Model file for the job. Use its own axes, mm. Face numbers are marked on the shaded views. A direction names the side the tool comes from. Round coordinates to 2 decimals unless told otherwise and drop trailing zeros. Order: outer loops, then holes, each group sorted by start corner. A loop starts at its lowest first (then second) coordinate and runs counter-clockwise, first axis right, second up. Notation, with made-up numbers: (6, -6.75) -> (52, -6.75) arc R29 cw to (52, 20.25) -> close; hole circle Ø8 at (-5.75, 12). An arc over 180 degrees is marked (long way). Put each result on its own line as item: value. Start each with the question number.
Q1. Cut at D-D, the plane z = 5. List the corners of the cut face in (x, y), and give its area (3 significant figures).
Q2. Cut at A-A, the plane z = 0. List the corners of the cut face in (x, y), and give its area (4 significant figures).
Q3. Flat gauge pins, fed straight in: P1, Ø5, axis at x = -10, z = 1.5, coming from the -Y side; P2, Ø2, axis at x = -5, z = 1.5, coming from the +Y side; P3, Ø4, axis at x = -18, y = -1, coming from the -Z side. Where does each tip first touch, or does it go through?
Q4. Probe L1, parallel to X at y = -4.25, z = -1.5; L2, parallel to X at y = -1.5, z = -3; L3, parallel to Y at x = -9.5, z = -1. List the from-to ranges inside material, lowest first.
Q5. Cut at C-C, the plane x = -6. List the corners of the cut face in (y, z).
Q6. Cut at B-B, the plane y = 0. List the corners of the cut face in (x, z), and give its area (4 significant figures).
Q7. 3-axis set-ups, long thin cutter, end or side, ignore diameter. For the marked faces 1 and 2: which of +Z, -Z, +X, -X, +Y, -Y reach the whole face in a straight line?
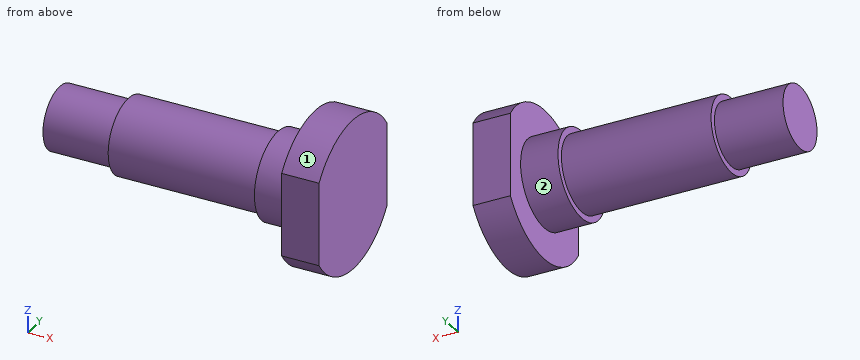
from build123d import *

# Parameters (mm, degrees)
BOSS_EXTRUDE1_DEPTH = 3
BOSS_EXTRUDE2_DEPTH = 15
BOSS_EXTRUDE3_DEPTH = 20.5
BOSS_EXTRUDE4_DEPTH = 3


with BuildPart() as part:
    # Sketch2 → Boss-Extrude1 (new body)
    with BuildSketch(Plane(origin=(0, 0, 0), x_dir=(0, 0, -1), z_dir=(1, 0, 0))):
        with BuildLine():
            Line((-3.31662479, 5), (3.31662479, 5))
            ThreePointArc((3.31662479, 5), (6, 0), (3.31662479, -5))
            Line((3.31662479, -5), (-3.31662479, -5))
            ThreePointArc((-3.31662479, -5), (-6, 0), (-3.31662479, 5))
        make_face()
    extrude(amount=BOSS_EXTRUDE1_DEPTH)

    # Sketch2_4 → Boss-Extrude2 (add)
    # profile 1 of 2: a face of its own
    with BuildSketch(Plane(origin=(0, 0, 0), x_dir=(0, 0, -1), z_dir=(1, 0, 0))):
        with BuildLine():
            ThreePointArc((3, 0), (0, 3), (-3, 0))
            ThreePointArc((-3, 0), (0, -3), (3, 0))
        make_face()
        with BuildLine():
            ThreePointArc((2.5, 0), (0, -2.5), (-2.5, 0))
            ThreePointArc((-2.5, 0), (0, 2.5), (2.5, 0))
        make_face(mode=Mode.SUBTRACT)
    # profile 2 of 2: a face of its own
    with BuildSketch(Plane(origin=(0, 0, 0), x_dir=(0, 0, -1), z_dir=(1, 0, 0))):
        with BuildLine():
            ThreePointArc((3, 0), (0, 3), (-3, 0))
            ThreePointArc((-3, 0), (0, -3), (3, 0))
        make_face()
        with BuildLine():
            ThreePointArc((2.5, 0), (0, -2.5), (-2.5, 0))
            ThreePointArc((-2.5, 0), (0, 2.5), (2.5, 0))
        make_face(mode=Mode.SUBTRACT)
    extrude(amount=-BOSS_EXTRUDE2_DEPTH)

    # Sketch2_5 → Boss-Extrude3 (add)
    with BuildSketch(Plane(origin=(0, 0, 0), x_dir=(0, 0, -1), z_dir=(1, 0, 0))):
        with BuildLine():
            ThreePointArc((2.5, 0), (0, 2.5), (-2.5, 0))
            ThreePointArc((-2.5, 0), (0, -2.5), (2.5, 0))
        make_face()
    extrude(amount=-BOSS_EXTRUDE3_DEPTH)

    # Sketch2_6 → Boss-Extrude4 (add)
    # profile 1 of 2: a face of its own
    with BuildSketch(Plane(origin=(0, 0, 0), x_dir=(0, 0, -1), z_dir=(1, 0, 0))):
        with BuildLine():
            ThreePointArc((3.5, 0), (0, 3.5), (-3.5, 0))
            ThreePointArc((-3.5, 0), (0, -3.5), (3.5, 0))
        make_face()
        with BuildLine():
            ThreePointArc((3, 0), (0, -3), (-3, 0))
            ThreePointArc((-3, 0), (0, 3), (3, 0))
        make_face(mode=Mode.SUBTRACT)
    # profile 2 of 2: a face of its own
    with BuildSketch(Plane(origin=(0, 0, 0), x_dir=(0, 0, -1), z_dir=(1, 0, 0))):
        with BuildLine():
            ThreePointArc((3.5, 0), (0, 3.5), (-3.5, 0))
            ThreePointArc((-3.5, 0), (0, -3.5), (3.5, 0))
        make_face()
        with BuildLine():
            ThreePointArc((3, 0), (0, -3), (-3, 0))
            ThreePointArc((-3, 0), (0, 3), (3, 0))
        make_face(mode=Mode.SUBTRACT)
    extrude(amount=-BOSS_EXTRUDE4_DEPTH)


solid = part.part
Ans:
1. outline: (0, -3.32) -> (3, -3.32) -> (3, 3.32) -> (0, 3.32) -> close
1. area: 19.9 mm^2
2. outline: (-20.5, -2.5) -> (-15, -2.5) -> (-15, -3) -> (-3, -3) -> (-3, -3.5) -> (0, -3.5) -> (0, -5) -> (3, -5) -> (3, 5) -> (0, 5) -> (0, 3.5) -> (-3, 3.5) -> (-3, 3) -> (-15, 3) -> (-15, 2.5) -> (-20.5, 2.5) -> close
2. area: 150.5 mm^2
3. P1: stops at y = -3
3. P2: stops at y = 2.96
3. P3: stops at z = -2.5
4. L1: x = 0 to 3
4. L2: x = -3 to 3
4. L3: y = -2.83 to 2.83
5. outline: circle Ø6 at (0, 0)
6. outline: (-20.5, -2.5) -> (-15, -2.5) -> (-15, -3) -> (-3, -3) -> (-3, -3.5) -> (0, -3.5) -> (0, -6) -> (3, -6) -> (3, 6) -> (0, 6) -> (0, 3.5) -> (-3, 3.5) -> (-3, 3) -> (-15, 3) -> (-15, 2.5) -> (-20.5, 2.5) -> close
6. area: 156.5 mm^2
7. face 1: +Z, +X, -X
7. face 2: -X
